Could you check a few things on this model? Use its own coordinates, in mm. A direction names the side the tool comes from. Give positions to 0.01 mm unless a question says otherwise; leave off trailing zeros. Loops run counter-clockwise (first coordinate to the right, second up) from the corner with the lowest first, then second, coordinate; pieces in that order, holes last. Notation, with made-up numbers: M 32,-9 L 40,-9 A32 cw 40,20 Z; hole C 3.25,59 d8. An arc over 180 degrees is marked long. Write each question's results on one line, items separated by ' | '. Start each with the question number.
from build123d import *

# Parameters (mm, degrees)
F1_DEPTH = 15


with BuildPart() as f1:
    # F0 (on Top) → F1 (new body)
    with BuildSketch(Plane.XY):
        with BuildLine():
            ThreePointArc((-17.1188699738, 7.52961819), (-5.85, 0), (-17.1188699738, -7.52961819))
            ThreePointArc((-17.1188699738, -7.52961819), (-19.7211173139, -7.011999011), (-22.3233646539, -7.52961819))
            ThreePointArc((-22.3233646539, -7.52961819), (-23.1351588042, -9.4894626373), (-21.1753143568, -10.3012567875))
            ThreePointArc((-21.1753143568, -10.3012567875), (-19.7211173139, -10.011999011), (-18.2669202709, -10.3012567875))
            ThreePointArc((-18.2669202709, -10.3012567875), (-10.6560319472, -10.6367465732), (-4.6062271062, -6.006623912))
            ThreePointArc((-4.6062271062, -6.006623912), (-2.85, 0), (-4.6062271062, 6.006623912))
            ThreePointArc((-4.6062271062, 6.006623912), (-10.6560319472, 10.6367465732), (-18.2669202709, 10.3012567875))
            ThreePointArc((-18.2669202709, 10.3012567875), (-19.7211173139, 10.011999011), (-21.1753143568, 10.3012567875))
            ThreePointArc((-21.1753143568, 10.3012567875), (-23.1351588042, 9.4894626373), (-22.3233646539, 7.52961819))
            ThreePointArc((-22.3233646539, 7.52961819), (-19.7211173139, 7.011999011), (-17.1188699738, 7.52961819))
        make_face()
        with BuildLine():
            ThreePointArc((-4.6062271062, 6.006623912), (-2.85, 0), (-4.6062271062, -6.006623912))
            ThreePointArc((-4.6062271062, -6.006623912), (-1.7984188449, -4.9538623094), (0, -7.3534005739))
            Line((0, -7.3534005739), (0, 0))
            Line((0, 0), (0, 7.3534005739))
            ThreePointArc((0, 7.3534005739), (-1.7984188449, 4.9538623094), (-4.6062271062, 6.006623912))
        make_face()
        with BuildLine():
            Line((0, 19.5), (0, 7.3534005739))
            Line((0, 7.3534005739), (0, 0))
            Line((0, 0), (3, 0))
            Line((3, 0), (3, 19.5))
            Line((3, 19.5), (5.5145750444, 20.1128965303))
            Line((5.5145750444, 20.1128965303), (5.4993545889, 19.4431964866))
            Line((5.4993545889, 19.4431964866), (8.0139296333, 20.0560930169))
            Line((8.0139296333, 20.0560930169), (7.9987091777, 19.3863929732))
            Line((7.9987091777, 19.3863929732), (10.5132842221, 19.9992895035))
            Line((10.5132842221, 19.9992895035), (10.4980637666, 19.3295894599))
            Line((10.4980637666, 19.3295894599), (13.012638811, 19.9424859902))
            Line((13.012638811, 19.9424859902), (12.9974183554, 19.2727859465))
            Line((12.9974183554, 19.2727859465), (15.5119933999, 19.8856824768))
            Line((15.5119933999, 19.8856824768), (15.4967729443, 19.2159824331))
            Line((15.4967729443, 19.2159824331), (18.0113479887, 19.8288789634))
            Line((18.0113479887, 19.8288789634), (17.9961275332, 19.1591789197))
            Line((17.9961275332, 19.1591789197), (20.5107025776, 19.77207545))
            Line((20.5107025776, 19.77207545), (20.495482122, 19.1023754063))
            ThreePointArc((20.495482122, 19.1023754063), (22.7516069101, 19.2212850643), (25, 19))
            add(Edge.make_bspline(
                [(3, 22.5), (8, 22.5), (16.9649489174, 21.8239376647), (24.4, 20.55), (25, 19)],
                knots=[0, 0, 0, 0, 0.5871428907, 1, 1, 1, 1], degree=3))
            ThreePointArc((3, 22.5), (0.8786796564, 21.6213203436), (0, 19.5))
        make_face()
        with BuildLine():
            Line((0, 0), (0, -7.3534005739))
            Line((0, -7.3534005739), (0, -19.5))
            ThreePointArc((0, -19.5), (0.8786796564, -21.6213203436), (3, -22.5))
            add(Edge.make_bspline(
                [(3, -22.5), (8, -22.5), (16.9649489174, -21.8239376647), (24.4, -20.55), (25, -19)],
                knots=[0, 0, 0, 0, 0.5871428907, 1, 1, 1, 1], degree=3))
            ThreePointArc((25, -19), (22.7516069101, -19.2212850643), (20.495482122, -19.1023754063))
            Line((20.495482122, -19.1023754063), (20.5107025776, -19.77207545))
            Line((20.5107025776, -19.77207545), (17.9961275332, -19.1591789197))
            Line((17.9961275332, -19.1591789197), (18.0113479887, -19.8288789634))
            Line((18.0113479887, -19.8288789634), (15.4967729443, -19.2159824331))
            Line((15.4967729443, -19.2159824331), (15.5119933999, -19.8856824768))
            Line((15.5119933999, -19.8856824768), (12.9974183554, -19.2727859465))
            Line((12.9974183554, -19.2727859465), (13.012638811, -19.9424859902))
            Line((13.012638811, -19.9424859902), (10.4980637666, -19.3295894599))
            Line((10.4980637666, -19.3295894599), (10.5132842221, -19.9992895035))
            Line((10.5132842221, -19.9992895035), (7.9987091777, -19.3863929732))
            Line((7.9987091777, -19.3863929732), (8.0139296333, -20.0560930169))
            Line((8.0139296333, -20.0560930169), (5.4993545889, -19.4431964866))
            Line((5.4993545889, -19.4431964866), (5.5145750444, -20.1128965303))
            Line((5.5145750444, -20.1128965303), (3, -19.5))
            Line((3, -19.5), (3, 0))
            Line((3, 0), (0, 0))
        make_face()
    extrude(amount=F1_DEPTH)


solid = f1.part
1) If we section it at B-B on y = 0: Write out the boundary of the cut face in (x, z).
2) Please list where these lines run through material, in increasing order: line 1 (Y direction, x = -14, z = 4.25); line 2 (X direction, y = 0, z = 11); line 3 (Y direction, x = -2.5, z = 2.25). Write a range as from..to.
3) Thinking about a two-plate mould opening in Y: for faces 1 (the face through (-10.76, -10.67, 7.4)), 2 (the face through (14.272, -19.584, 7.395)), 3 (the face through (-1, 0, 0)), 4 (the face through (-23.147, -9.459, 7.395)), which applies, pulls with the +Y half, pulls with the -Y half, needs draft (parallel to the pull), parting line crosses it, or undercut?
4) If we section it at D-D on y = -18: Write out the boundary of the cut face in (x, z), plus the area to 3 significant figures.
5) I'm going to push flat-ended pins straight in: P1, Ø1, axis at y = -13, z = 5.5, coming from the -X side; P2, Ø4, axis at x = 17, z = 4.5, coming from the +Y side; P3, Ø2, axis at x = -11.5, z = 1.5, coming from the -Y side; P4, Ø4, axis at y = 10.5, z = 8.5, coming from the -X side. Where does each tip first touch, or does it pass through?
6) Which directions (+Z, -Z, +X, -X, +Y, -Y) give clear straight access to the entire face, cutting with the end or side of a thin tool? Please do faces 5 (the face through (-19.7, 10.012, 7.395)), 6 (the face through (0, -13, 7)), 7 (the face through (6.739, 19.745, 7.395)).
7) If we section it at A-A on x = -14: Write out the boundary of the cut face in (y, z).
8) If we section it at C-C on x = -6.5: Write out the boundary of the cut face in (y, z), plus the area to 3 significant figures.
Calculated:
1) outline: M -5.85,0 L 3,0 L 3,15 L -5.85,15 Z
2) line 1: y = -11.15..-8.15, 8.15..11.15 | line 2: x = -5.85..3 | line 3: y = -4.85..4.85
3) face 1: pulls with the -Y half | face 2: undercut | face 3: needs draft | face 4: undercut
4) outline: M 0,0 L 3,0 L 3,15 L 0,15 Z | area: 45.0 mm2
5) P1: stops at x = 0 | P2: stops at y = 21.85 | P3: stops at y = -11.05 | P4: stops at x = -23.25
6) face 5: +Z, -Z, +Y | face 6: +Z, -Z, -Y | face 7: +Z, -Z
7) outline: M -11.15,0 L -8.15,0 L -8.15,15 L -11.15,15 Z; M 8.15,0 L 11.15,0 L 11.15,15 L 8.15,15 Z
8) outline: M -8.25,0 L -3.19,0 L -3.19,15 L -8.25,15 Z; M 3.19,0 L 8.25,0 L 8.25,15 L 3.19,15 Z | area: 152 mm2
